```python
from build123d import *

# Parameters (mm, degrees)
F2_R = 3
F3_R = 5
F4_R = 5


with BuildPart() as f1:
    # F0 (on Front) → F1 (revolve)
    with BuildSketch(Plane.XZ):
        Polygon((0, -32.151528), (0, -27.619155), (-23.653328, -27.619155), (-23.653328, 42.915918), (-29.885342, 42.915918), (-59.948665, -41.193824), (-55.434137, -41.193824), (-27.90243, 35.55081), (-27.90243, -32.151528), (-23.370055, -32.151528), align=None)
    revolve(axis=Axis((0, 0, -29.885341), (0, 0, -1)))

    # F2
    f2_edges = [f1.edges().sort_by_distance(p)[0] for p in [
        (29.885342, 0, 42.915918),
        (23.653328, 0, 42.915918),
    ]]
    fillet(f2_edges, radius=F2_R)

    # F3
    f3_edges = [f1.edges().sort_by_distance(p)[0] for p in [
        (23.653328, 0, -27.619155),
    ]]
    fillet(f3_edges, radius=F3_R)

    # F4
    f4_edges = [f1.edges().sort_by_distance(p)[0] for p in [
        (27.90243, 0, -32.151528),
    ]]
    fillet(f4_edges, radius=F4_R)


solid = f1.part
```
Read the model definition and answer for the solid it produces. Units are mm, in the model's axes. A direction names the side the tool comes from. Coordinates: 2 decimals unless noted, no trailing zeros. Order: outer loops, then holes, each group sorted by start corner. A loop starts at its lowest first (then second) coordinate and runs counter-clockwise, first axis right, second up. Notation, with made-up numbers: (88, 5) - (146, 5) arc R23 ccw to (146, 43) - close; hole circle Ø11 at (19.25, 24). An arc over 180 degrees is marked (long way). Answer as a JSON object with one key per item and string values. Group by question number.
Item 1: Section D-D (z = 29) is taken. Give the vertices of the cut face in (x, y) (1 decimal).
Item 2: Section A-A (x = 0) is taken. Give the vertices of the cut face in (y, z), plus the area to 3 significant figures.
Item 3: Consider probe 1 along Y at (x, z) = (0, 7.5); probe 2 along Y at (x, z) = (-25.5, -5); probe 3 along Y at (x, z) = (0, -7.5). Determine where each line is inside the solid, lowest interval first. Write a range as from..to.
Item 4: Section B-B (z = 20) is taken. Give the vertices of the cut face in (x, y), plus the area to 3 significant figures.
Item 5: The mould has two halves that part along X. Classify faces 3 (the face through (0, 0, -27.619)), 4 (the face through (-17.98, -34.56, 17.54)), 5 (the face through (-53, -17, -41.194)), 6 (the face through (-22.561, 7.105, 9.086)): +X half, -X half, draft (parallel to the pull), parting line (faces both ways), or undercut.
Item 6: Flat-ended cylindrical pins translate along their axes: P1, Ø1, axis at x = -8, z = -13.5, coming from the +Y side; P2, Ø10, axis at x = -40.5, z = -28, coming from the +Y side; P3, Ø4, axis at y = -38.5, z = -1, coming from the -X side. Find the tip coordinate at first contact, or state that the pin passes through.
Item 7: A tool of negligible diameter and unlimited length cuts with its end or side. For faces 1 (the face through (-25, 10, 42.916)), 2 (the face through (0, 0, -32.152)), from which of +Z, -Z, +X, -X, +Y, -Y can it reach the whole face along a straight path? Write none if from no direction.
Results are:
{
 "1": {"outline": "circle Ø69.7 at (0, 0); circle Ø55.8 at (0, 0); hole circle Ø60.5 at (0, 0); hole circle Ø47.3 at (0, 0)"},
 "2": {"outline": "(-59.95, -41.19) - (-55.43, -41.19) - (-27.9, 35.55) - (-27.9, -27.15) arc R5 ccw to (-22.9, -32.15) - (22.9, -32.15) arc R5 ccw to (27.9, -27.15) - (27.9, 35.55) - (55.43, -41.19) - (59.95, -41.19) - (30.6, 40.93) arc R3 ccw to (27.77, 42.92) - (26.65, 42.92) arc R3 ccw to (23.65, 39.92) - (23.65, -22.62) arc R5 cw to (18.65, -27.62) - (-18.65, -27.62) arc R5 cw to (-23.65, -22.62) - (-23.65, 39.92) arc R3 ccw to (-26.65, 42.92) - (-27.77, 42.92) arc R3 ccw to (-30.6, 40.93) - close", "area": "1,600 mm^2"},
 "3": {"probe 1": "y = -42.54..-37.97, -27.9..-23.65, 23.65..27.9, 37.97..42.54", "probe 2": "y = -39.5..-33.94, -11.33..11.33, 33.94..39.5", "probe 3": "y = -47.91..-43.35, -27.9..-23.65, 23.65..27.9, 43.35..47.91"},
 "4": {"outline": "circle Ø76.15 at (0, 0); circle Ø55.8 at (0, 0); hole circle Ø66.96 at (0, 0); hole circle Ø47.31 at (0, 0)", "area": "1,720 mm^2"},
 "5": {"face 3": "undercut", "face 4": "parting line", "face 5": "draft", "face 6": "undercut"},
 "6": {"P1": "stops at y = 49.6", "P2": "stops at y = 42.92", "P3": "stops at x = -27.56"},
 "7": {"face 1": "+Z, +X, -X, +Y, -Y", "face 2": "-Z"}
}
